Design review of the part built by this model. Coordinates are the model's own, in mm. Face numbers are marked on the shaded views. A direction names the side the tool comes from. Coordinates: 2 decimals unless noted, no trailing zeros. Loops run counter-clockwise (first coordinate to the right, second up) from the corner with the lowest first, then second, coordinate; pieces in that order, holes last.
Q1. Add section A-A on y = 72. Give the boundary of the cut face in (x, z).
Q2. For P1, Ø4, axis at x = -51.5, z = -76.5, coming from the +Y side; P2, Ø5, axis at x = -55, y = 23.5, coming from the +Z side; P3, Ø1, axis at x = -4.5, z = -45, coming from the +Y side, all flat-tipped, find the tip position at first contact; note any pin that passes through.
Q3. Wall thickness on probe 1 along Z at (x, y) = (-88.5, 57.5); probe 2 along X at (y, z) = (82, -70.5); probe 3 along Y at (x, z) = (-104, -11): over which ranges is each line inside the solid? List them lowest first.
Q4. Add section C-C on y = 81.5. Give the boundary of the cut face in (x, z), and give its area (3 significant figures).
Q5. Machinability: for the marked faces 1, 2 and 3, which of the approach directions +Z, -Z, +X, -X, +Y, -Y give a long, thin tool a straight path to every point of the face, cutting with its end or side? Answer none if there is none.
Q6. Draft analysis for pull direction X (two halves, no side actions). For the marked faces 4, 5 and 6, state which applies: released by +X, released by -X, zero draft, split by the parting line, or undercut.
Q7. Add section D-D on z = -34. Give the boundary of the cut face in (x, y).
Q8. Add section B-B on x = -31.5. Give the boundary of the cut face in (y, z), and give its area (3 significant figures).
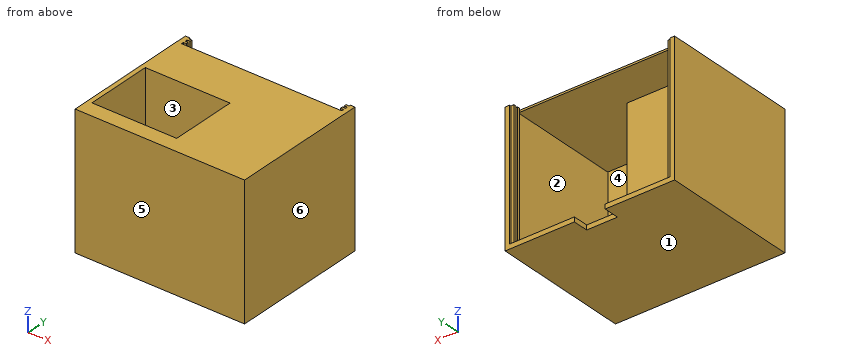
Autodesk Inventor part; units mm, degrees
ref_plane "YZ Plane" through (0, 0, 0) normal (1, 0, 0) x (0, 1, 0)
ref_plane "XZ Plane" through (0, 0, 0) normal (0, 1, 0) x (-1, 0, 0)
ref_plane "XY Plane" through (0, 0, 0) normal (0, 0, 1) x (1, 0, 0)
sketch "Sketch12" plane through (0, 0, 0) normal (0, 1, 0) x (-1, 0, 0)
  line L0 (0, 0) -> (110, 0)
  line L1 (110, 0) -> (110, -86)
  line L2 (110, -86) -> (0, -86)
  line L3 (0, -86) -> (0, 0)
  dimension "d23" = 110
  dimension "d24" = 86
extrude "Extrusion6" add sketch "Sketch12" along normal blind 10
sketch "Sketch13" plane through (0, 10, 0) normal (0, 1, 0) x (1, 0, 0)
  line L0 (0, 0) -> (0, 86)
  line L1 (-110, 0) -> (0, 0)
  line L2 (0, 86) -> (-110, 86)
  line L3 (-110, 86) -> (-110, 0)
  line L4 (-107, 43) -> (-107, 83)
  line L5 (-107, 83) -> (-107, 0)
  line L6 (-107, 83) -> (-3, 83)
  line L7 (-3, 0) -> (-3, 83)
extrude "Extrusion7" add sketch "Sketch13" along normal blind 80 contours L1 L7 L6 L4 L5 L3 L2 L0
sketch "Sketch14" plane through (-107, 10, -83) normal (0, 0, 1) x (1, 0, 0)
  line L0 (0, 80) -> (104, 80)
  line L1 (62, 80) -> (42, 80)
  line L2 (42, 80) -> (42, 70)
  line L3 (42, 70) -> (62, 70)
  line L4 (62, 70) -> (62, 80)
  point P0 (107, -10)
  dimension "d33" = 20
  dimension "d34" = 10
  dimension "d35" = 20
extrude "Extrusion8" cut sketch "Sketch14" against normal through all
sketch "Sketch15" plane through (-107, 10, 0) normal (1, 0, 0) x (0, 0, -1)
  line L0 (0, 80) -> (83, 80)
  line L1 (41.5, 79) -> (83, 79)
  line L2 (83, 0) -> (83, 80)
  line L3 (83, 79) -> (0, 79)
  line L4 (0, 0) -> (0, 80)
  line L5 (0, 79) -> (0, 77.5)
  line L6 (0, 77.5) -> (83, 77.5)
  line L7 (0, 76) -> (83, 76)
  line L8 (83, 76) -> (83, 74.5)
  line L9 (83, 74.5) -> (0, 74.5)
  line L10 (0, 76) -> (0, 74.5)
  line L11 (83, 79) -> (83, 77.5)
  point P0 (0, -10)
  dimension "d39" = 1.5
  dimension "d40" = 1.5
  dimension "d41" = 1.5
extrude "Extrusion9" add sketch "Sketch15" along normal blind 2 contours L3 L1 L2 L6 L4 | L7 L2 L9 L4
sketch "Sketch16" plane through (-3, 10, -83) normal (-1, 0, 0) x (0, 0, 1)
  line L0 (0, 80) -> (83, 80)
  line L1 (41.5, 79) -> (0, 79)
  line L2 (0, 0) -> (0, 80)
  line L3 (0, 79) -> (83, 79)
  line L4 (83, 0) -> (83, 80)
  line L5 (83, 79) -> (83, 77.5)
  line L6 (83, -10) -> (83, 80)
  line L7 (83, 77.5) -> (0, 77.5)
  line L8 (0, 77.5) -> (0, 79)
  line L9 (0, 76) -> (83, 76)
  line L10 (83, 76) -> (83, 74.5)
  line L11 (83, 74.5) -> (0, 74.5)
  line L12 (0, 74.5) -> (0, 76)
  point P0 (0, 74.5)
  point P1 (0, 76)
  dimension "d45" = 1.5
  dimension "d46" = 1.5
  dimension "d47" = 1.5
extrude "Extrusion10" add sketch "Sketch16" along normal blind 2 contours L1 L3 L4 L7 L2 | L9 L4 L11 L2
sketch "Sketch17" plane through (-107, 10, 0) normal (1, 0, 0) x (0, 0, -1)
  line L0 (83, 74.5) -> (0, 74.5)
  line L1 (0, 0) -> (0, 74.5)
  line L2 (0, 43.5) -> (83, 43.5)
  line L3 (83, 0) -> (83, 74.5)
  line L4 (83, 43.5) -> (83, 46)
  line L5 (83, 46) -> (0, 45.9998)
  line L6 (0, 45.9998) -> (0, 43.5)
  point P0 (0, -10)
  dimension "d50" = 31
  dimension "d51" = 2.5
extrude "Extrusion11" add sketch "Sketch17" along normal blind 55 contours L3 L2 L1 L5
sketch "Sketch18" plane through (-107, 84.5, 0) normal (1, 0, 0) x (0, 0, -1)
  line L0 (0, -84.5) -> (0, 5.5)
  line L1 (0, -28.5002) -> (0, 0)
  line L2 (0, -1.5292) -> (0, -28.5002)
  line L3 (0, -28.5002) -> (1.25, -28.5002)
  line L4 (0, -28.5002) -> (83, -28.5)
  line L5 (1.25, -28.5002) -> (1.25, -1.5292)
  line L6 (1.25, -1.5292) -> (0, -1.5292)
  dimension "d54" = 1.25
  dimension "d55" = 26.971
extrude "Extrusion12" add sketch "Sketch18" along normal up to surface (104 mm away)
sketch "Sketch19" plane through (-52, 55.9998, -1.25) normal (0, -1, 0) x (1, 0, 0)
  line L0 (0, 0) -> (0, 1.25)
  line L1 (0, 1.25) -> (49, 1.25)
  line L2 (0, 1.25) -> (49, 1.25)
  line L3 (49, 1.25) -> (49, 0)
  line L4 (49, 1.25) -> (49, 0)
  line L5 (0, 0) -> (49, 0)
  line L6 (0, 1.25) -> (0, 0)
  line L7 (0, -81.75) -> (0, 0)
  line L8 (0, 0) -> (49, 0)
  point P0 (52, 1.2502)
extrude "Extrusion13" add sketch "Sketch19" along normal up to surface (45.9998 mm away)
sketch "Sketch20" plane through (-110, 0, 0) normal (0, 0, 1) x (1, 0, 0)
  point P0 (110, 0)
properties part number "circuit casing"
Entries:
1. outline: (-110, -86) - (0, -86) - (0, 0) - (-110, 0) - close; hole (-107, -83) - (-3, -83) - (-3, -1.25) - (-107, -1.25) - close
2. P1: stops at y = 56
2. P2: stops at z = -83
2. P3: stops at y = 89
3. probe 1: z = -86 to -83, -1.25 to 0
3. probe 2: x = -110 to -107, -3 to 0
3. probe 3: y = 0 to 10, 53.5 to 56
4. outline: (-110, -86) - (-65, -86) - (-65, -83) - (-107, -83) - (-107, -1.25) - (-3, -1.25) - (-3, -83) - (-45, -83) - (-45, -86) - (0, -86) - (0, 0) - (-110, 0) - close
4. area: 898 mm2
5. face 1: -Z, +X, -X, +Y, -Y
5. face 2: none
5. face 3: +Z
6. face 4: undercut
6. face 5: zero draft
6. face 6: released by +X
7. outline: (-110, 0) - (0, 0) - (0, 90) - (-3, 90) - (-3, 89) - (-5, 89) - (-5, 87.5) - (-3, 87.5) - (-3, 86) - (-5, 86) - (-5, 84.5) - (-3, 84.5) - (-3, 10) - (-107, 10) - (-107, 53.5) - (-52, 53.5) - (-52, 56) - (-107, 56) - (-107, 84.5) - (-105, 84.5) - (-105, 86) - (-107, 86) - (-107, 87.5) - (-105, 87.5) - (-105, 89) - (-107, 89) - (-107, 90) - (-110, 90) - close
8. outline: (0, -86) - (90, -86) - (90, -83) - (10, -83) - (10, -1.25) - (82.97, -1.25) - (82.97, 0) - (0, 0) - close
8. area: 1,190 mm2
